Geometry check sheet. Reference: the model listing, model coordinates, mm. Face numbers are marked on the shaded views. A direction names the side the tool comes from. Coordinates: 2 decimals unless noted, no trailing zeros. Order: outer loops, then holes, each group sorted by start corner. A loop starts at its lowest first (then second) coordinate and runs counter-clockwise, first axis right, second up.
```python
from build123d import *

# Parameters (mm, degrees)
BOSS_EXTRUDE1_DEPTH = 2.5
BOSS_EXTRUDE2_DEPTH = 50
CUT_EXTRUDE1_REACH  = 94.879


with BuildPart() as part:
    # Sketch1 → Boss-Extrude1 (new body)
    with BuildSketch(Plane(origin=(0, 0, 0), x_dir=(1, 0, 0), z_dir=(0, 1, 0))):
        Polygon((20, -17.5), (35, -17.5), (35, 17.5), (-35, 17.5), (-35, -17.5), (-20, -17.5), (-20, -67.5), (20, -67.5), align=None)
    extrude(amount=BOSS_EXTRUDE1_DEPTH)

    # Sketch3 → Boss-Extrude2 (add)
    with BuildSketch(Plane(origin=(0, 2.5, 0), x_dir=(1, 0, 0), z_dir=(0, 1, 0))):
        Polygon((-35, 17.5), (-32.5, 17.5), (32.5, 17.5), (35, 17.5), (35, -2.5), (32.5, -2.5), (32.5, 15), (1.25, 15), (1.25, -2.5), (-1.25, -2.5), (-1.25, 15), (-32.5, 15), (-32.5, -2.5), (-35, -2.5), align=None)
    extrude(amount=BOSS_EXTRUDE2_DEPTH)

    # Sketch4 → Cut-Extrude1 (cut, up to next)
    with BuildSketch(Plane(origin=(1.25, 0, 0), x_dir=(0, 0, -1), z_dir=(1, 0, 0)), mode=Mode.PRIVATE) as cut_extrude1_sk1:
        Polygon((15, 2.5), (-2.5, 52.5), (-2.5, 2.5), align=None)
    cut_extrude1_tool1 = extrude(cut_extrude1_sk1.sketch, amount=-CUT_EXTRUDE1_REACH, mode=Mode.PRIVATE) & part.part
    add(cut_extrude1_tool1.solids().sort_by_distance((1.25, 19.166667, -3.333333))[0], mode=Mode.SUBTRACT)


solid = part.part
```
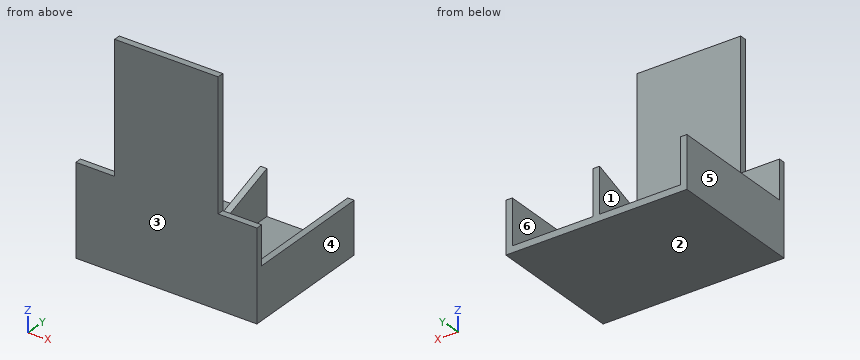
Item 1: Thickness scan on line 1 along X through (y, z) = (43, -1.5); line 2 along Y through (x, z) = (14.5, 9.5); line 3 along Z through (x, y) = (-20.5, 34.5). Record the ranges inside material, lowest first.
Item 2: Release check for a two-part mould opening along X. For the marked faces 3, 4, 5 and 6 record: pulls with the +X half, pulls with the -X half, needs draft (parallel to the pull), parting line crosses it, or undercut.
Item 3: Depth check by flat-ended pin: P1, Ø0.8, axis at x = 24, y = 1, coming from the +Z side; P2, Ø3, axis at y = 1, z = 54.5, coming from the -X side; P3, Ø8, axis at x = -13.5, y = 20, coming from the +Z side; P4, Ø3, axis at x = -1, z = 25, coming from the -Y side. Enter the tip coordinate at first touch or a pass-through.
Item 4: Sectioned sample at C-C (x = 9). Record the cut outline in (y, z), and give its area (4 significant figures).
Item 5: Sectioned sample at D-D (z = 3.5). Record the cut outline in (x, y), and give its area (3 significant figures).
Item 6: Tool access check on the marked faces 1 and 2. Record the directions out of +Z, -Z, +X, -X, +Y, -Y that give a thin tool (end or side, any length) a straight path to the whole face; none if there is none.
Item 7: Sectioned sample at B-B (y = 18.5). Record the cut outline in (x, z).
Item 8: Sectioned sample at A-A (z = -12). Record the cut outline in (x, y), and give its area (3 significant figures).
Geometry check:
1. line 1: x = -35 to -32.5, -1.25 to 1.25, 32.5 to 35
1. line 2: y = 0 to 2.5
1. line 3: z = -17.5 to -15
2. face 3: needs draft
2. face 4: pulls with the +X half
2. face 5: pulls with the -X half
2. face 6: undercut
3. P1: stops at z = 17.5
3. P2: stops at x = -20
3. P3: stops at z = -15
3. P4: stops at y = 0
4. outline: (0, -17.5) - (52.5, -17.5) - (52.5, -15) - (2.5, -15) - (2.5, 67.5) - (0, 67.5) - close
4. area: 337.5 mm2
5. outline: (-35, 0) - (35, 0) - (35, 2.5) - (-35, 2.5) - close
5. area: 175 mm2
6. face 1: +Z, +Y
6. face 2: -Z, +X, -X, +Y, -Y
7. outline: (-35, -17.5) - (35, -17.5) - (35, 2.5) - (32.5, 2.5) - (32.5, -15) - (1.25, -15) - (1.25, -9.4) - (-1.25, -9.4) - (-1.25, -15) - (-32.5, -15) - (-32.5, 2.5) - (-35, 2.5) - close
8. outline: (-35, 0) - (35, 0) - (35, 52.5) - (32.5, 52.5) - (32.5, 2.5) - (-32.5, 2.5) - (-32.5, 52.5) - (-35, 52.5) - close; (-1.25, 11.07) - (1.25, 11.07) - (1.25, 52.5) - (-1.25, 52.5) - close
8. area: 529 mm2
